```python
from build123d import *

# Parameters (mm, degrees)
SKETCH1_R      = 12.7
EXTRUDE1_DEPTH = 12.7
SKETCH2_R      = 4.7625
SKETCH2_R_2    = 3.8735
EXTRUDE2_START = 0.889
SKETCH4_R      = 4.7625
EXTRUDE2_DEPTH = 0.889


with BuildPart() as part:
    # Sketch1 → Extrude1 (new, symmetric)
    with BuildSketch(Plane(origin=(0, 0, 0), x_dir=(0, 0, -1), z_dir=(1, 0, 0))):
        Circle(SKETCH1_R)
    extrude(amount=EXTRUDE1_DEPTH, both=True)

    # Sweep1: sweep along a path in Sketch3
    with BuildLine(Plane(origin=(0, 0, 0), x_dir=(0, 0, -1), z_dir=(1, 0, 0))) as sweep1_path:
        Line((12.7, -12.7), (-38.1, -12.7))
        ThreePointArc((-38.1, -12.7), (-60.550640303, -21.999359697), (-69.85, -44.45))
        Line((-69.85, -44.45), (-69.85, -63.5))
    # Sketch2 → Sweep1 (sweep)
    with BuildSketch(Plane.XY.offset(-12.7)):
        with Locations((0, -12.7)):
            Circle(SKETCH2_R)
        with Locations((0, -12.7)):
            Circle(SKETCH2_R_2, mode=Mode.SUBTRACT)
    sweep(path=sweep1_path.line)

    # Sketch4 → Extrude2 (add)
    with BuildSketch(Plane.XY.offset(-12.7).offset(EXTRUDE2_START)):
        with Locations(Location((0, -12.7, 0), (0, 0, 90))):
            Circle(SKETCH4_R)
    extrude(amount=-EXTRUDE2_DEPTH)

    # Sketch5 → Revolve1 (revolve)
    with BuildSketch(Plane(origin=(0, 0, 0), x_dir=(0, 0, -1), z_dir=(1, 0, 0))):
        Polygon((-10.16, 0), (-31.115, 0), (-31.115, 1.5875), (-23.462887774, 1.5875), (-22.225, 4.0259), (-10.16, 4.0259), align=None)
    revolve(axis=Axis((0, 0, 31.115), (0, 0, 1)))


solid = part.part
```
Geometry check sheet. Reference: the model listing, model coordinates, mm. A direction names the side the tool comes from. Give positions to 0.01 mm unless a question says otherwise; leave off trailing zeros. Order: outer loops, then holes, each group sorted by start corner. A loop starts at its lowest first (then second) coordinate and runs counter-clockwise, first axis right, second up.
1. Access from +Z, -Z, +X, -X, +Y, -Y to the whole of each face (thin tool, end or side, straight path). Record for faces 5 (the face through (-12.7, 0, 0)), 6 (the face through (0, 0, 31.115)), 7 (the face through (-1.03, -54.11, 65.2)), 8 (the face through (0.1, -12.7, 0.1)), 9 (the face through (1.55, -0.34, 27.24)).
2. Release check for a two-part mould opening along Y. For faces 1 (the face through (0, -13, -11.811)), 2 (the face through (-4, -63.5, 69)), 3 (the face through (12.7, 0, 0)), 4 (the face through (-0.84, -16.48, 13.49)) record: pulls with the +Y half, pulls with the -Y half, needs draft (parallel to the pull), parting line crosses it, or undercut.
3. Gauge pin test, flat ends, axial feed: pin 1 Ø5 at (x, z) = (-6, 35.5) entering from +Y; pin 2 Ø2.5 at (x, y) = (-2, -11.5) entering from +Z; pin 3 Ø12 at (x, y) = (6, -50) entering from -Z; pin 4 Ø3 at (x, z) = (-8, 48) entering from -Y. Record the tip position at first contact, or that the pin passes through.
4. Section check C-C, the plane y = 0. Enter the section's corners in (x, z) (1 decimal).
5. Section check A-A, the plane z = 28.5. Enter the section's corners in (x, y) (1 decimal).
6. Thickness scan on L1, parallel to Y at x = 0, z = 18.5; L2, parallel to Y at x = 0, z = 24; L3, parallel to X at y = -12.7, z = 18. Record the ranges inside material, lowest first.
7. Section check B-B, the plane z = 0. Enter the section's corners in (x, y) (1 decimal).
Values follow:
1. face 5: +Z, -Z, -X, +Y, -Y
1. face 6: +Z, +X, -X, +Y
1. face 7: -Y
1. face 8: none
1. face 9: +Z
2. face 1: undercut
2. face 2: pulls with the -Y half
2. face 3: needs draft
2. face 4: undercut
3. pin 1: stops at y = -9.47
3. pin 2: stops at z = 55.54
3. pin 3: stops at z = 65.09
3. pin 4: passes through
4. outline: (-12.7, -12.7) - (12.7, -12.7) - (12.7, 12.7) - (4, 12.7) - (4, 22.2) - (1.6, 23.5) - (1.6, 31.1) - (-1.6, 31.1) - (-1.6, 23.5) - (-4, 22.2) - (-4, 12.7) - (-12.7, 12.7) - close
5. outline: circle Ø9.5 at (0, -12.7); circle Ø3.2 at (0, 0); hole circle Ø7.7 at (0, -12.7)
6. L1: y = -17.46 to -16.57, -8.83 to -7.94, -4.03 to 4.03
6. L2: y = -17.46 to -16.57, -8.83 to -7.94, -1.59 to 1.59
6. L3: x = -4.76 to -3.87, 3.87 to 4.76
7. outline: (-12.7, -12.7) - (-4.8, -12.7) arc R4.8 ccw to (4.8, -12.7) - (12.7, -12.7) - (12.7, 12.7) - (-12.7, 12.7) - close; hole (-3.9, -12.7) arc R3.9 ccw to (3.9, -12.7) - close
